Design review of the part shown in the three views and the two pictorial views. Dimensions are in mm from the part's minimum x, y and z. A direction names the side the tool comes from. Round coordinates to 2 decimals unless told otherwise and drop trailing zeros. Order: outer loops, then holes, each group sorted by start corner. A loop starts at its lowest first (then second) coordinate and runs counter-clockwise, first axis right, second up. Notation, with made-up numbers: (-3.75, 33.5) -> (7.25, 33.5) arc R32 cw to (7.25, 62.5) -> close; hole circle Ø1 at (47.5, 33.25). An arc over 180 degrees is marked (long way). Put each result on its own line as item: value. Start each with the question number.
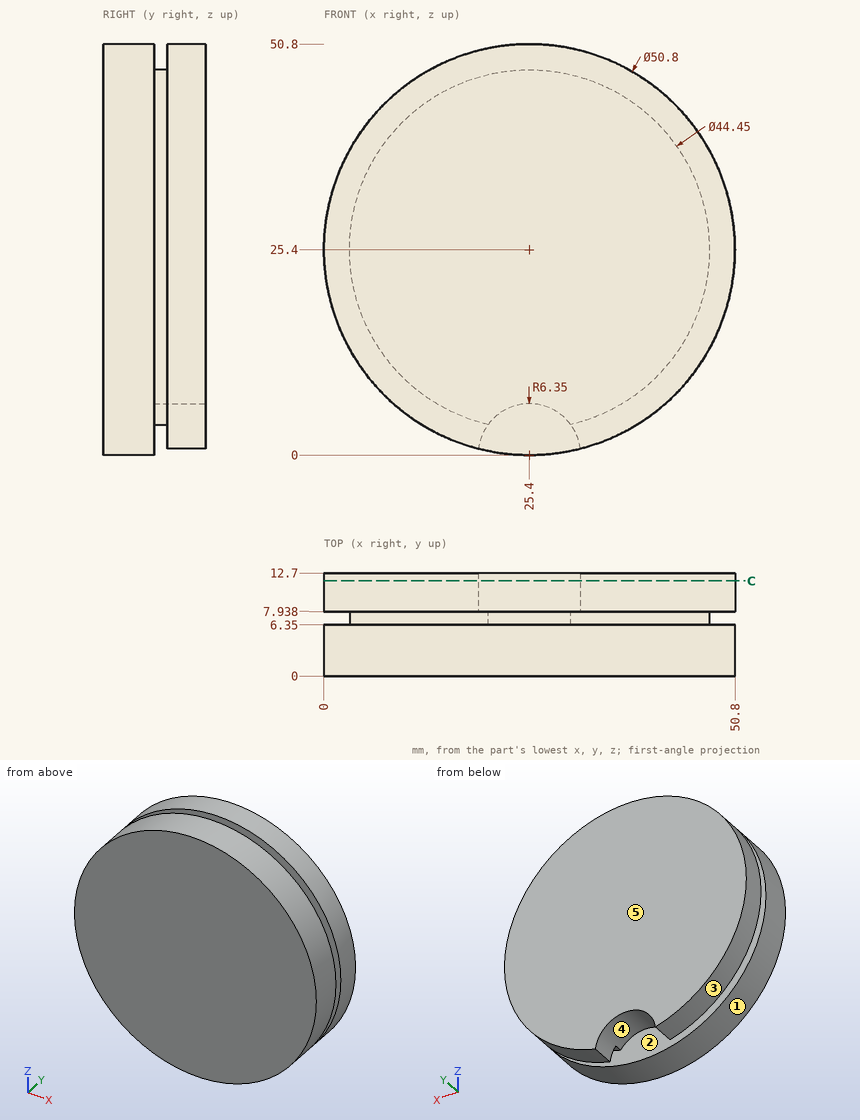
Q1. Clearance check with flat-ended pins moving along their axes: pin 1 Ø4 at (y, z) = (4, 30) entering from -X; pin 2 Ø1 at (x, y) = (5.5, 10.5) entering from -Z (1 decimal); pin 3 Ø2 at (x, y) = (15.5, 4.5) entering from -Z. State where each tip first meets the part, or that it passes through.
Q2. For the marked faces 1 and 2, list the 3-axis set-ups (+Z, -Z, +X, -X, +Y, -Y) from which the entire face can be reached by the end or side of a thin tool; tool diameter is ignored.
Q3. Draft analysis for pull direction X (two halves, no side actions). For the marked faces 3, 4 and 5, state which applies: +X half, -X half, draft (parallel to the pull), parting line (faces both ways), or undercut.
Q4. Wall thickness on probe 1 along X at (y, z) = (7.5, 13.5); probe 2 along Z at (x, y) = (32, 10); probe 3 along X at (y, z) = (6, 23): over which ranges is each line inside the solid? List them lowest first. Write a range as [from, to].
Q5. Take a section at C-C on y = 11.75. Give the boundary of the cut face in (x, z), and give its area (3 significant figures).
Calculated:
1. pin 1: stops at x = 0.13
1. pin 2: stops at z = 9
1. pin 3: stops at z = 1.61
2. face 1: +Y, -Y
2. face 2: none
3. face 3: parting line
3. face 4: undercut
3. face 5: draft
4. probe 1: x = [6.63, 44.17]
4. probe 2: z = [0.87, 49.93]
4. probe 3: x = [0.11, 50.69]
5. outline: (19.1, 0.79) arc R6.35 cw to (31.7, 0.79) arc R25.4 ccw (long way) to start
5. area: 1,970 mm²
